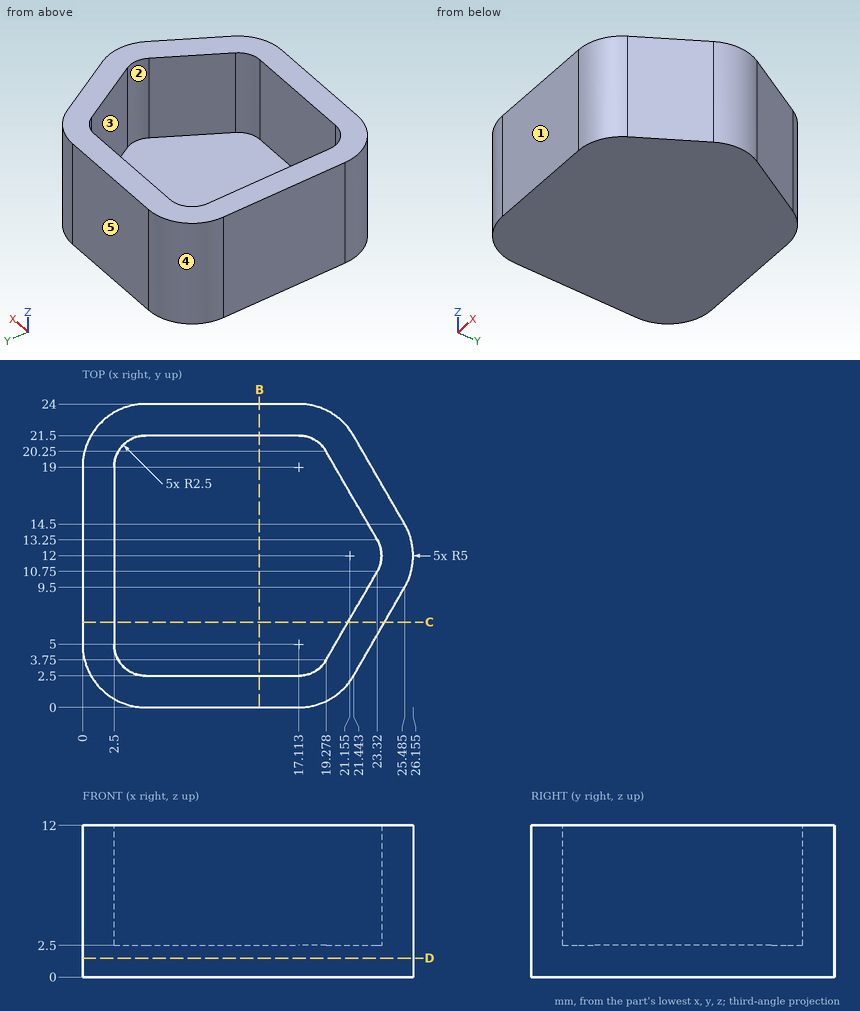
The figure shows three views and two pictorial views of one solid part (mm, origin at its lowest corner). Answer the questions. A direction names the side the tool comes from. Give positions to 0.01 mm unless a question says otherwise; leave off trailing zeros. Write each loop counter-clockwise with the first axis right and the second up, starting at its lowest first coordinate (ties: lowest second). Pieces come first, ordered by that corner, then holes.
Q1. A tool of negligible diameter and unlimited length cuts with its end or side. For the marked faces 1 and 2, from which of +Z, -Z, +X, -X, +Y, -Y can it reach the whole face along a straight path? Write none if from no direction.
Answer:
face 1: +Z, -Z, +X, -X, -Y
face 2: +Z
Q2. For a pull along X with two mould halves and no side action, classify the marked faces 3, 4 and 5 as released by +X, released by -X, zero draft, split by the parting line, or undercut.
Answer:
face 3: undercut
face 4: released by -X
face 5: zero draft
Q3. The part is cut by section C-C on y = 6.75. Give the vertices of the cut face in (x, z).
Answer:
outline: (0, 0) - (23.9, 0) - (23.9, 12) - (21.01, 12) - (21.01, 2.5) - (2.5, 2.5) - (2.5, 12) - (0, 12) - close
Q4. Straight lines are drawn through the part: L1, parallel to X at y = 12, z = 6.5 (1 decimal); L2, parallel to Y at x = 11.5, z = 6; L3, parallel to Z at x = 13.5, y = 12.5. For each, find the intervals that lie inside material, in ascending order.
Answer:
L1: x = 0 to 2.5, 23.7 to 26.2
L2: y = 0 to 2.5, 21.5 to 24
L3: z = 0 to 2.5
Q5. Given pin 1 (2 mm diameter, centred on x = 19.5, z = 4, fed in from -Y); pin 2 (8 mm diameter, centred on x = 7, y = 7, fed in from +Z); pin 3 (1 mm diameter, centred on x = 23.5, z = 8.5, fed in from +Y) (1 decimal), each flat-ended and moving along its own axis, determine where each tip first touches the part or whether it passes through.
Answer:
pin 1: stops at y = 0.2
pin 2: stops at z = 2.5
pin 3: stops at y = 18.8
Q6. The part is cut by section D-D on z = 1.5. Give the vertices of the cut face in (x, y) (1 decimal).
Answer:
outline: (0, 5) arc R5 ccw to (5, 0) - (17.1, 0) arc R5 ccw to (21.4, 2.5) - (25.5, 9.5) arc R5 ccw to (25.5, 14.5) - (21.4, 21.5) arc R5 ccw to (17.1, 24) - (5, 24) arc R5 ccw to (0, 19) - close
Q7. The part is cut by section B-B on x = 14. Give the vertices of the cut face in (y, z).
Answer:
outline: (0, 0) - (24, 0) - (24, 12) - (21.5, 12) - (21.5, 2.5) - (2.5, 2.5) - (2.5, 12) - (0, 12) - close
